Here's how the part is built. I have some questions about the finished solid (model axes, mm). A direction names the side the tool comes from. Round coordinates to 2 decimals unless told otherwise and drop trailing zeros. Write each loop counter-clockwise with the first axis right and the second up, starting at its lowest first coordinate (ties: lowest second). Pieces come first, ordered by that corner, then holes. Notation, with made-up numbers: (69, 84) -> (101, 84) arc R31 cw to (101, 121) -> close; hole circle Ø9 at (26.25, -33.5). An arc over 180 degrees is marked (long way). Answer in a Markdown table with one row per item. Add a question column.
from build123d import *

# Parameters (mm, degrees)
ESQUISSE1_W             = 24
ESQUISSE1_H             = 20
BOSS_EXTRU_1_DEPTH      = 1.5
ESQUISSE2_W             = 4.9
ESQUISSE2_H             = 3
BOSS_EXTRU_2_DEPTH      = 1.5
ENL_V_MAT_EXTRU_1_REACH = 25.372
ESQUISSE3_R             = 1.5


with BuildPart() as part:
    # Esquisse1 → Boss.-Extru.1 (new body)
    with BuildSketch(Plane.XY):
        with Locations((0, 10)):
            Rectangle(ESQUISSE1_W, ESQUISSE1_H)
    extrude(amount=BOSS_EXTRU_1_DEPTH)

    # Esquisse2 → Boss.-Extru.2 (add)
    with BuildSketch(Plane.XY):
        with Locations((7.05, -1.5)):
            Rectangle(ESQUISSE2_W, ESQUISSE2_H)
        with Locations((-7.05, -1.5)):
            Rectangle(ESQUISSE2_W, ESQUISSE2_H)
    extrude(amount=BOSS_EXTRU_2_DEPTH)

    # Esquisse3 → Enlèv. mat.-Extru.1 (cut, up to next)
    with BuildSketch(Plane.XY.offset(1.5), mode=Mode.PRIVATE) as enl_v_mat_extru_1_sk1:
        with Locations((-7, 3)):
            Circle(ESQUISSE3_R)
    enl_v_mat_extru_1_tool1 = extrude(enl_v_mat_extru_1_sk1.sketch, amount=-ENL_V_MAT_EXTRU_1_REACH, mode=Mode.PRIVATE) & part.part
    # Esquisse3 → Enlèv. mat.-Extru.1 (cut, up to next)
    with BuildSketch(Plane.XY.offset(1.5), mode=Mode.PRIVATE) as enl_v_mat_extru_1_sk2:
        with Locations((-2.5, 3)):
            Circle(ESQUISSE3_R)
    enl_v_mat_extru_1_tool2 = extrude(enl_v_mat_extru_1_sk2.sketch, amount=-ENL_V_MAT_EXTRU_1_REACH, mode=Mode.PRIVATE) & part.part
    # Esquisse3 → Enlèv. mat.-Extru.1 (cut, up to next)
    with BuildSketch(Plane.XY.offset(1.5), mode=Mode.PRIVATE) as enl_v_mat_extru_1_sk3:
        with Locations((2, 3)):
            Circle(ESQUISSE3_R)
    enl_v_mat_extru_1_tool3 = extrude(enl_v_mat_extru_1_sk3.sketch, amount=-ENL_V_MAT_EXTRU_1_REACH, mode=Mode.PRIVATE) & part.part
    # Esquisse3 → Enlèv. mat.-Extru.1 (cut, up to next)
    with BuildSketch(Plane.XY.offset(1.5), mode=Mode.PRIVATE) as enl_v_mat_extru_1_sk4:
        with Locations((6.5, 3)):
            Circle(ESQUISSE3_R)
    enl_v_mat_extru_1_tool4 = extrude(enl_v_mat_extru_1_sk4.sketch, amount=-ENL_V_MAT_EXTRU_1_REACH, mode=Mode.PRIVATE) & part.part
    # Esquisse3 → Enlèv. mat.-Extru.1 (cut, up to next)
    with BuildSketch(Plane.XY.offset(1.5), mode=Mode.PRIVATE) as enl_v_mat_extru_1_sk5:
        with Locations((-2.5, 7.5)):
            Circle(ESQUISSE3_R)
    enl_v_mat_extru_1_tool5 = extrude(enl_v_mat_extru_1_sk5.sketch, amount=-ENL_V_MAT_EXTRU_1_REACH, mode=Mode.PRIVATE) & part.part
    # Esquisse3 → Enlèv. mat.-Extru.1 (cut, up to next)
    with BuildSketch(Plane.XY.offset(1.5), mode=Mode.PRIVATE) as enl_v_mat_extru_1_sk6:
        with Locations((2, 7.5)):
            Circle(ESQUISSE3_R)
    enl_v_mat_extru_1_tool6 = extrude(enl_v_mat_extru_1_sk6.sketch, amount=-ENL_V_MAT_EXTRU_1_REACH, mode=Mode.PRIVATE) & part.part
    # Esquisse3 → Enlèv. mat.-Extru.1 (cut, up to next)
    with BuildSketch(Plane.XY.offset(1.5), mode=Mode.PRIVATE) as enl_v_mat_extru_1_sk7:
        with Locations((6.5, 7.5)):
            Circle(ESQUISSE3_R)
    enl_v_mat_extru_1_tool7 = extrude(enl_v_mat_extru_1_sk7.sketch, amount=-ENL_V_MAT_EXTRU_1_REACH, mode=Mode.PRIVATE) & part.part
    # Esquisse3 → Enlèv. mat.-Extru.1 (cut, up to next)
    with BuildSketch(Plane.XY.offset(1.5), mode=Mode.PRIVATE) as enl_v_mat_extru_1_sk8:
        with Locations((-2.5, 12)):
            Circle(ESQUISSE3_R)
    enl_v_mat_extru_1_tool8 = extrude(enl_v_mat_extru_1_sk8.sketch, amount=-ENL_V_MAT_EXTRU_1_REACH, mode=Mode.PRIVATE) & part.part
    # Esquisse3 → Enlèv. mat.-Extru.1 (cut, up to next)
    with BuildSketch(Plane.XY.offset(1.5), mode=Mode.PRIVATE) as enl_v_mat_extru_1_sk9:
        with Locations((2, 12)):
            Circle(ESQUISSE3_R)
    enl_v_mat_extru_1_tool9 = extrude(enl_v_mat_extru_1_sk9.sketch, amount=-ENL_V_MAT_EXTRU_1_REACH, mode=Mode.PRIVATE) & part.part
    # Esquisse3 → Enlèv. mat.-Extru.1 (cut, up to next)
    with BuildSketch(Plane.XY.offset(1.5), mode=Mode.PRIVATE) as enl_v_mat_extru_1_sk10:
        with Locations((6.5, 12)):
            Circle(ESQUISSE3_R)
    enl_v_mat_extru_1_tool10 = extrude(enl_v_mat_extru_1_sk10.sketch, amount=-ENL_V_MAT_EXTRU_1_REACH, mode=Mode.PRIVATE) & part.part
    # Esquisse3 → Enlèv. mat.-Extru.1 (cut, up to next)
    with BuildSketch(Plane.XY.offset(1.5), mode=Mode.PRIVATE) as enl_v_mat_extru_1_sk11:
        with Locations((-2.5, 16.5)):
            Circle(ESQUISSE3_R)
    enl_v_mat_extru_1_tool11 = extrude(enl_v_mat_extru_1_sk11.sketch, amount=-ENL_V_MAT_EXTRU_1_REACH, mode=Mode.PRIVATE) & part.part
    # Esquisse3 → Enlèv. mat.-Extru.1 (cut, up to next)
    with BuildSketch(Plane.XY.offset(1.5), mode=Mode.PRIVATE) as enl_v_mat_extru_1_sk12:
        with Locations((2, 16.5)):
            Circle(ESQUISSE3_R)
    enl_v_mat_extru_1_tool12 = extrude(enl_v_mat_extru_1_sk12.sketch, amount=-ENL_V_MAT_EXTRU_1_REACH, mode=Mode.PRIVATE) & part.part
    # Esquisse3 → Enlèv. mat.-Extru.1 (cut, up to next)
    with BuildSketch(Plane.XY.offset(1.5), mode=Mode.PRIVATE) as enl_v_mat_extru_1_sk13:
        with Locations((6.5, 16.5)):
            Circle(ESQUISSE3_R)
    enl_v_mat_extru_1_tool13 = extrude(enl_v_mat_extru_1_sk13.sketch, amount=-ENL_V_MAT_EXTRU_1_REACH, mode=Mode.PRIVATE) & part.part
    # Esquisse3 → Enlèv. mat.-Extru.1 (cut, up to next)
    with BuildSketch(Plane.XY.offset(1.5), mode=Mode.PRIVATE) as enl_v_mat_extru_1_sk14:
        with Locations((-7, 7.5)):
            Circle(ESQUISSE3_R)
    enl_v_mat_extru_1_tool14 = extrude(enl_v_mat_extru_1_sk14.sketch, amount=-ENL_V_MAT_EXTRU_1_REACH, mode=Mode.PRIVATE) & part.part
    # Esquisse3 → Enlèv. mat.-Extru.1 (cut, up to next)
    with BuildSketch(Plane.XY.offset(1.5), mode=Mode.PRIVATE) as enl_v_mat_extru_1_sk15:
        with Locations((-7, 12)):
            Circle(ESQUISSE3_R)
    enl_v_mat_extru_1_tool15 = extrude(enl_v_mat_extru_1_sk15.sketch, amount=-ENL_V_MAT_EXTRU_1_REACH, mode=Mode.PRIVATE) & part.part
    # Esquisse3 → Enlèv. mat.-Extru.1 (cut, up to next)
    with BuildSketch(Plane.XY.offset(1.5), mode=Mode.PRIVATE) as enl_v_mat_extru_1_sk16:
        with Locations((-7, 16.5)):
            Circle(ESQUISSE3_R)
    enl_v_mat_extru_1_tool16 = extrude(enl_v_mat_extru_1_sk16.sketch, amount=-ENL_V_MAT_EXTRU_1_REACH, mode=Mode.PRIVATE) & part.part
    add(enl_v_mat_extru_1_tool1.solids().sort_by_distance((-7, 3, 1.5))[0], mode=Mode.SUBTRACT)
    add(enl_v_mat_extru_1_tool2.solids().sort_by_distance((-2.5, 3, 1.5))[0], mode=Mode.SUBTRACT)
    add(enl_v_mat_extru_1_tool3.solids().sort_by_distance((2, 3, 1.5))[0], mode=Mode.SUBTRACT)
    add(enl_v_mat_extru_1_tool4.solids().sort_by_distance((6.5, 3, 1.5))[0], mode=Mode.SUBTRACT)
    add(enl_v_mat_extru_1_tool5.solids().sort_by_distance((-2.5, 7.5, 1.5))[0], mode=Mode.SUBTRACT)
    add(enl_v_mat_extru_1_tool6.solids().sort_by_distance((2, 7.5, 1.5))[0], mode=Mode.SUBTRACT)
    add(enl_v_mat_extru_1_tool7.solids().sort_by_distance((6.5, 7.5, 1.5))[0], mode=Mode.SUBTRACT)
    add(enl_v_mat_extru_1_tool8.solids().sort_by_distance((-2.5, 12, 1.5))[0], mode=Mode.SUBTRACT)
    add(enl_v_mat_extru_1_tool9.solids().sort_by_distance((2, 12, 1.5))[0], mode=Mode.SUBTRACT)
    add(enl_v_mat_extru_1_tool10.solids().sort_by_distance((6.5, 12, 1.5))[0], mode=Mode.SUBTRACT)
    add(enl_v_mat_extru_1_tool11.solids().sort_by_distance((-2.5, 16.5, 1.5))[0], mode=Mode.SUBTRACT)
    add(enl_v_mat_extru_1_tool12.solids().sort_by_distance((2, 16.5, 1.5))[0], mode=Mode.SUBTRACT)
    add(enl_v_mat_extru_1_tool13.solids().sort_by_distance((6.5, 16.5, 1.5))[0], mode=Mode.SUBTRACT)
    add(enl_v_mat_extru_1_tool14.solids().sort_by_distance((-7, 7.5, 1.5))[0], mode=Mode.SUBTRACT)
    add(enl_v_mat_extru_1_tool15.solids().sort_by_distance((-7, 12, 1.5))[0], mode=Mode.SUBTRACT)
    add(enl_v_mat_extru_1_tool16.solids().sort_by_distance((-7, 16.5, 1.5))[0], mode=Mode.SUBTRACT)


solid = part.part
Item 1: If we mould it in two halves opening along X, with no side actions, what happens to faces 1 (the flat face through (-11, 0, 1)), 2 (the cylindrical face through (5.3, 11.1, 0.8)), 3 (the flat face through (9.5, -2, 1)), 4 (the cylindrical face through (-1.81, 1.67, 0.76))? For each: pulls with the +X half, pulls with the -X half, needs draft (parallel to the pull), parting line crosses it, or undercut.
Item 2: If we section it at B-B on y = 7.5: Please give me the cut outline in (x, z).
Item 3: For P1, Ø5, axis at x = 6.5, y = 8.5, coming from the +Z side; P2, Ø0.8, axis at x = 10.5, z = 0.5, coming from the -Y side; P3, Ø0.8, axis at y = -2, z = 0.5, coming from the +X side, each with a flat end and sliding along its axis, tell me the tip position at first contact or that it passes through.
Item 4: I need wall thicknesses on line 1 along Y through (x, z) = (-7, 0.4); line 2 along Y through (x, z) = (2, 0.6); line 3 along X through (y, z) = (6.25, 0.25). Which ranges of each line are inside material? Lowest first, please. Write a range as from..to.
Item 5: If we section it at D-D on x = 10: Please give me the cut outline in (y, z).
Item 6: If we section it at C-C on z = 0.3: Give the number of separate pieces and of enclosed holes in the cut face, then the cut area to 3 significant figures.
Item 7: On a 3-axis mill with a long thin cutter (end or side, diameter ignored), from which of +Z, -Z, +X, -X, +Y, -Y can I reach the whole of each face in a straight line? I mean faces 5 (the cylindrical face through (-2.825, 6.036, 0.76)), 6 (the flat face through (-4.6, -2, 1)). Say none if no direction works.
Item 8: If we section it at A-A on x = -2.5: Please give me the cut outline in (y, z), then the cut area to 3 significant figures.
Results list:
| question | item | result |
|---|---|---|
| 1 | face 1 | needs draft |
| 1 | face 2 | undercut |
| 1 | face 3 | pulls with the +X half |
| 1 | face 4 | undercut |
| 2 | outline | (-12, 0) -> (-8.5, 0) -> (-8.5, 1.5) -> (-12, 1.5) -> close; (-5.5, 0) -> (-4, 0) -> (-4, 1.5) -> (-5.5, 1.5) -> close; (-1, 0) -> (0.5, 0) -> (0.5, 1.5) -> (-1, 1.5) -> close; (3.5, 0) -> (5, 0) -> (5, 1.5) -> (3.5, 1.5) -> close; (8, 0) -> (12, 0) -> (12, 1.5) -> (8, 1.5) -> close |
| 3 | P1 | z = 1.5 |
| 3 | P2 | y = 0 |
| 3 | P3 | x = 9.5 |
| 4 | line 1 | -3..1.5, 4.5..6, 9..10.5, 13.5..15, 18..20 |
| 4 | line 2 | 0..1.5, 4.5..6, 9..10.5, 13.5..15, 18..20 |
| 4 | line 3 | -12..-7.83, -6.17..-3.33, -1.67..1.17, 2.83..5.67, 7.33..12 |
| 5 | outline | (0, 0) -> (20, 0) -> (20, 1.5) -> (0, 1.5) -> close |
| 6 | separate pieces | 1 |
| 6 | enclosed holes | 16 |
| 6 | area | 396 mm² |
| 7 | face 5 | +Z, -Z |
| 7 | face 6 | +Z, -Z, -Y |
| 8 | outline | (0, 0) -> (1.5, 0) -> (1.5, 1.5) -> (0, 1.5) -> close; (4.5, 0) -> (6, 0) -> (6, 1.5) -> (4.5, 1.5) -> close; (9, 0) -> (10.5, 0) -> (10.5, 1.5) -> (9, 1.5) -> close; (13.5, 0) -> (15, 0) -> (15, 1.5) -> (13.5, 1.5) -> close; (18, 0) -> (20, 0) -> (20, 1.5) -> (18, 1.5) -> close |
| 8 | area | 12.0 mm² |
